```python
from build123d import *

# Parameters (mm, degrees)
SKETCH001_W     = 30
SKETCH001_H     = 30
PAD_DEPTH       = 20
POCKET_DEPTH    = 4.5
POCKET001_DEPTH = 20
SKETCH004_R     = 3
HOLE001_DEPTH   = 30.001
SKETCH005_R     = 1.1049
HOLE002_DEPTH   = 9.336109
HOLE002_TIPS_R  = 1.1049
SKETCH_R        = 1.65
HOLE_DEPTH      = 20.001


with BuildPart() as part:
    # Sketch001 → Pad (new body)
    with BuildSketch(Plane.XY):
        with Locations((4.5, 0)):
            Rectangle(SKETCH001_W, SKETCH001_H)
    extrude(amount=PAD_DEPTH)

    # Sketch002 (on DatumPlane) → Pocket (cut)
    with BuildSketch(Plane(origin=(19.5, 0, 10), x_dir=(0, 1, 0), z_dir=(1, 0, 0))):
        with BuildLine():
            Line((-8.99, 6), (8.99, 6))
            ThreePointArc((11.067944, 3.523602), (10.606354, 5.246282), (8.99, 6))
            Line((11.067944, 3.523602), (9.69612, -4.256398))
            ThreePointArc((7.618176, -6), (8.974458, -5.506354), (9.69612, -4.256398))
            Line((-7.618176, -6), (7.618176, -6))
            ThreePointArc((-9.69612, -4.256398), (-8.974458, -5.506354), (-7.618176, -6))
            Line((-11.067944, 3.523602), (-9.69612, -4.256398))
            ThreePointArc((-8.99, 6), (-10.606354, 5.246282), (-11.067944, 3.523602))
        make_face()
    extrude(amount=-POCKET_DEPTH, mode=Mode.SUBTRACT)

    # Sketch003 (on DatumPlane) → Pocket001 (cut)
    with BuildSketch(Plane(origin=(19.5, 0, 10), x_dir=(0, 1, 0), z_dir=(1, 0, 0))):
        with BuildLine():
            Line((-7.1, 4.5), (7.1, 4.5))
            ThreePointArc((9.069616, 2.152704), (8.632089, 3.785575), (7.1, 4.5))
            Line((9.069616, 2.152704), (8.187981, -2.847296))
            ThreePointArc((6.218365, -4.5), (7.50394, -4.032089), (8.187981, -2.847296))
            Line((-6.218365, -4.5), (6.218365, -4.5))
            ThreePointArc((-8.187981, -2.847296), (-7.50394, -4.032089), (-6.218365, -4.5))
            Line((-9.069616, 2.152704), (-8.187981, -2.847296))
            ThreePointArc((-7.1, 4.5), (-8.632089, 3.785575), (-9.069616, 2.152704))
        make_face()
    extrude(amount=-POCKET001_DEPTH, mode=Mode.SUBTRACT)

    # Sketch004 (on DatumPlane) → Hole001 (cut, through all)
    with BuildSketch(Plane(origin=(19.5, 0, 10), x_dir=(0, 1, 0), z_dir=(1, 0, 0))):
        Circle(SKETCH004_R)
    extrude(amount=-HOLE001_DEPTH, mode=Mode.SUBTRACT)

    # Sketch005 (on DatumPlane) → Hole002 (cut)
    with BuildSketch(Plane(origin=(19.5, 0, 10), x_dir=(0, 1, 0), z_dir=(1, 0, 0))):
        with Locations((-12.495, 0)):
            Circle(SKETCH005_R)
        with Locations((12.495, 0)):
            Circle(SKETCH005_R)
    extrude(amount=-HOLE002_DEPTH, mode=Mode.SUBTRACT)

    # Hole002 tips → Hole002 tip 1 section 0
    with BuildSketch(Plane(origin=(10.163891, 0, 10), x_dir=(0, 1, 0), z_dir=(1, 0, 0)), mode=Mode.PRIVATE) as hole002_tip_1_s0:
        with Locations((-12.495, 0)):
            Circle(HOLE002_TIPS_R)
    loft([hole002_tip_1_s0.sketch, Vertex(9.5, -12.495, 10)], mode=Mode.SUBTRACT)

    # Hole002 tips → Hole002 tip 2 section 0
    with BuildSketch(Plane(origin=(10.163891, 0, 10), x_dir=(0, 1, 0), z_dir=(1, 0, 0)), mode=Mode.PRIVATE) as hole002_tip_2_s0:
        with Locations((12.495, 0)):
            Circle(HOLE002_TIPS_R)
    loft([hole002_tip_2_s0.sketch, Vertex(9.5, 12.495, 10)], mode=Mode.SUBTRACT)

    # Sketch (on DatumPlane) → Hole (cut, through all)
    with BuildSketch(Plane.XY.offset(20)):
        with Locations((-7.5, 12)):
            Circle(SKETCH_R)
        with Locations((7.5, 12)):
            Circle(SKETCH_R)
        with Locations((7.5, -12)):
            Circle(SKETCH_R)
        with Locations((-7.5, -12)):
            Circle(SKETCH_R)
    extrude(amount=-HOLE_DEPTH, mode=Mode.SUBTRACT)


solid = part.part
```
Geometry check sheet. Reference: the model listing, model coordinates, mm. A direction names the side the tool comes from. Coordinates: 2 decimals unless noted, no trailing zeros. Write each loop counter-clockwise with the first axis right and the second up, starting at its lowest first coordinate (ties: lowest second). Pieces come first, ordered by that corner, then holes. Notation, with made-up numbers: M 0,4 L 43,4 A8 ccw 43,15 Z; hole C 39.5,65 d2. An arc over 180 degrees is marked long. One line per item, written item: value. Start each with the question number.
(1) Tool access check on faces 5 (the face through (7, 0, 5.5)), 6 (the face through (-8.81, -13, 10.14)). Record the directions out of +Z, -Z, +X, -X, +Y, -Y that give a thin tool (end or side, any length) a straight path to the whole face; none if there is none.
(2) Sectioned sample at B-B, the plane x = -7.5. Enter the section's corners in (y, z).
(3) Scan lines: line 1 along X through (y, z) = (11, 17.5); line 2 along Z through (x, y) = (1.75, 2.5); line 3 along X through (y, z) = (12.75, 19.25). Record each from-to range of solid material in increasing order. Write a range as [from, to].
(4) Sectioned sample at A-A, the plane y = 0. Enter the section's corners in (x, z), and give its area (4 significant figures).
(5) Release check for a two-part mould opening along X. For faces 1 (the face through (-8.81, 11, 10.14)), 2 (the face through (14.9, -13.6, 10)), 3 (the face through (6.19, -13, 10.14)), 4 (the face through (-10.5, -4, 10)) record: released by +X, released by -X, zero draft, split by the parting line, or undercut.
(6) Sectioned sample at D-D, the plane x = -4.25. Enter the section's corners in (y, z).
(7) Sectioned sample at C-C, the plane z = 18. Enter the section's corners in (x, y).
(8) Depth check by flat-ended pin: pin 1 (1.8 mm diameter, centred on y = 12.495, z = 10, fed in from +X); pin 2 (7 mm diameter, centred on y = -1, z = 10.5, fed in from +X). Enter the tip coordinate at first touch or a pass-through.
Filled sheet:
1. face 5: +X
1. face 6: +Z, -Z
2. outline: M -15,0 L -13.65,0 L -13.65,20 L -15,20 Z; M -10.35,0 L 10.35,0 L 10.35,20 L -10.35,20 Z; M 13.65,0 L 15,0 L 15,20 L 13.65,20 Z; hole C 0,10 d6
3. line 1: [-10.5, -8.81], [-6.19, 6.19], [8.81, 19.5]
3. line 2: [0, 5.5], [14.5, 20]
3. line 3: [-10.5, -8.97], [-6.03, 6.03], [8.97, 19.5]
4. outline: M -10.5,0 L 19.5,0 L 19.5,4 L 15,4 L 15,5.5 L -0.5,5.5 L -0.5,7 L -10.5,7 Z; M -10.5,13 L -0.5,13 L -0.5,14.5 L 15,14.5 L 15,16 L 19.5,16 L 19.5,20 L -10.5,20 Z
4. area: 346.5 mm²
5. face 1: undercut
5. face 2: zero draft
5. face 3: undercut
5. face 4: released by -X
6. outline: M -15,0 L 15,0 L 15,20 L -15,20 Z; hole C 0,10 d6
7. outline: M -10.5,-15 L 19.5,-15 L 19.5,15 L -10.5,15 Z; hole C -7.5,-12 d3.3; hole C -7.5,12 d3.3; hole C 7.5,-12 d3.3; hole C 7.5,12 d3.3
8. pin 1: x = 10.04
8. pin 2: x = -0.5
